Source: CAD feature listing. Evaluate the final solid. Frame: model axes, mm. A direction names the side the tool comes from. Give positions to 0.01 mm unless a question says otherwise; leave off trailing zeros. Loops run counter-clockwise (first coordinate to the right, second up) from the corner with the lowest first, then second, coordinate; pieces in that order, holes last. Notation, with made-up numbers: (59.5, 29.5) -> (94.5, 29.5) arc R21 cw to (94.5, 68.5) -> close; hole circle Ø11 at (-28.75, 51). An arc over 180 degrees is marked (long way). Return JSON: item names as keys, results as strings. Group by question number.
```python
from build123d import *

# Parameters (mm, degrees)
SKETCH1_R           = 2.159
SKETCH1_W           = 6.35
SKETCH1_H           = 6.35
BOSS_EXTRUDE1_DEPTH = 6.35


with BuildPart() as part:
    # Sketch1 → Boss-Extrude1 (new body)
    with BuildSketch(Plane(origin=(0, 0, 0), x_dir=(1, 0, 0), z_dir=(0, 1, 0))):
        Polygon((-25.4, 76.2), (-47.875911854, 76.2), (-60.633073629, 76.2), (-42.466090347, -115.062), (-22.93356755, -115.062), (-22.93356755, -120.142), (-41.98356755, -120.142), (-41.332161775, -127), (-28.575, -127), (0, -127), (28.575, -127), (41.332161775, -127), (60.633073629, 76.2), (47.875911854, 76.2), (25.4, 76.2), (25.4, 0), (13.208, 0), (13.208, 57.15), (6.858, 57.15), (6.858, 0), (-6.858, 0), (-6.858, 57.15), (-13.208, 57.15), (-13.208, 0), (-25.4, 0), align=None)
        Polygon((-39.17295277, -82.578452823), (-39.773403679, -76.256905647), (-33.451856503, -75.656454737), (-32.851405593, -81.978001914), align=None, mode=Mode.SUBTRACT)
        with Locations(Location((-37.41723431, -67.485806976, 0), (0, 0, 270))):
            Circle(SKETCH1_R, mode=Mode.SUBTRACT)
        Polygon((-35.66151585, -52.393161128), (-35.061064941, -58.714708304), (-41.382612117, -59.315159214), (-41.983063027, -52.993612037), align=None, mode=Mode.SUBTRACT)
        Polygon((29.83293553, -113.756454737), (36.154482707, -114.356905647), (35.554031797, -120.678452823), (29.232484621, -120.078001914), align=None, mode=Mode.SUBTRACT)
        with Locations(Location((33.798313337, -105.585806976, 0), (0, 0, 270))):
            Circle(SKETCH1_R, mode=Mode.SUBTRACT)
        Polygon((37.763691145, -97.415159214), (31.442143968, -96.814708304), (32.042594878, -90.493161128), (38.364142054, -91.093612037), align=None, mode=Mode.SUBTRACT)
        Polygon((-50.786897864, 39.693161128), (-51.387348774, 46.014708304), (-45.065801597, 46.615159214), (-44.465350687, 40.293612037), align=None, mode=Mode.SUBTRACT)
        with Locations((-34.925, 43.307)):
            Rectangle(SKETCH1_W, SKETCH1_H, mode=Mode.SUBTRACT)
        with Locations(Location((-49.031179404, 54.785806976, 0), (0, 0, 270))):
            Circle(SKETCH1_R, mode=Mode.SUBTRACT)
        Polygon((-47.275460944, 69.878452823), (-46.675010035, 63.556905647), (-52.996557211, 62.956454737), (-53.597008121, 69.278001914), align=None, mode=Mode.SUBTRACT)
        with Locations(Location((-34.925, 54.991, 0), (0, 0, 270))):
            Circle(SKETCH1_R, mode=Mode.SUBTRACT)
        with Locations((-34.925, 66.675)):
            Rectangle(SKETCH1_W, SKETCH1_H, mode=Mode.SUBTRACT)
        with Locations((34.925, 43.307)):
            Rectangle(SKETCH1_W, SKETCH1_H, mode=Mode.SUBTRACT)
        Polygon((45.065801597, 46.615159214), (51.387348774, 46.014708304), (50.786897864, 39.693161128), (44.465350687, 40.293612037), align=None, mode=Mode.SUBTRACT)
        with Locations(Location((34.925, 54.991, 0), (0, 0, 270))):
            Circle(SKETCH1_R, mode=Mode.SUBTRACT)
        with Locations((34.925, 66.675)):
            Rectangle(SKETCH1_W, SKETCH1_H, mode=Mode.SUBTRACT)
        with Locations(Location((49.031179404, 54.785806976, 0), (0, 0, 270))):
            Circle(SKETCH1_R, mode=Mode.SUBTRACT)
        Polygon((52.996557211, 62.956454737), (46.675010035, 63.556905647), (47.275460944, 69.878452823), (53.597008121, 69.278001914), align=None, mode=Mode.SUBTRACT)
    extrude(amount=BOSS_EXTRUDE1_DEPTH)


solid = part.part
```
1) Cut plane D-D on z = 16.5. Return loops of the section in (x, y).
2) Reachability of faces 5 (the face through (-22.934, 3, 118)), 6 (the face through (43, 3, -76.2)), 7 (the face through (-35, 3, -69.85)) from +Z, -Z, +X, -X, +Y, -Y: full face, straight path, thin tool, end or side. Return the list, or none.
3) Cut plane B-B on x = -21. Return loops of the section in (y, z).
4) Cut plane A-A on z = -10. Return loops of the section in (x, y), then the cut area to 3 significant figures.
5) Contact query for flat-ended pins moving along their axis: P1, Ø7, axis at x = -49.03, z = -54.79, coming from the -Y side; P2, Ø3, axis at y = 3, z = -42, coming from the +X side; P3, Ø3, axis at x = 19, y = 4, coming from the -Z side; P4, Ø3, axis at y = 3, z = -45, coming from the -X side. Output: stop coordinate, or through.
6) Material intervals for line 1 (Z direction, x = -24.5, y = 5.75); line 2 (X direction, y = 2.25, z = -23.5); line 3 (X direction, y = 4.75, z = -51), sorted ascending.
7) Cut plane C-C on y = 1. Count the separate pieces of the cut face and the enclosed holes in it, then the cut area to 3 significant figures.
8) Mould query, pull axis X, two halves, no side actions, for faces 1 (the face through (-47.6, 3.1, -56.4)), 2 (the face through (-1, 3, 127)), 3 (the face through (-41.662, 3.131, 123.523)), 4 (the face through (38.07, 3.13, 94.21)). Classes: released by +X, released by -X, zero draft, split by the parting line, or undercut.
Calculated:
{
 "1": {"outline": "(-51.83, 0) -> (51.83, 0) -> (51.83, 6.35) -> (-51.83, 6.35) -> close"},
 "2": {"face 5": "-X, +Y, -Y", "face 6": "-Z, +X, -X, +Y, -Y", "face 7": "+Y, -Y"},
 "3": {"outline": "(0, 0) -> (6.35, 0) -> (6.35, 127) -> (0, 127) -> close"},
 "4": {"outline": "(-54.35, 0) -> (-25.4, 0) -> (-25.4, 6.35) -> (-54.35, 6.35) -> close; (-13.21, 0) -> (-6.86, 0) -> (-6.86, 6.35) -> (-13.21, 6.35) -> close; (6.86, 0) -> (13.21, 0) -> (13.21, 6.35) -> (6.86, 6.35) -> close; (25.4, 0) -> (54.35, 0) -> (54.35, 6.35) -> (25.4, 6.35) -> close", "area": "448 mm2"},
 "5": {"P1": "y = 0", "P2": "x = 57.53", "P3": "z = 0", "P4": "x = -57.81"},
 "6": {"line 1": "0 to 115.06, 120.14 to 127", "line 2": "-55.63 to -25.4, -13.21 to -6.86, 6.86 to 13.21, 25.4 to 55.63", "line 3": "-58.24 to -25.4, -13.21 to -6.86, 6.86 to 13.21, 25.4 to 58.24"},
 "7": {"separate pieces": "1", "enclosed holes": "18", "area": "16,900 mm2"},
 "8": {"face 1": "undercut", "face 2": "zero draft", "face 3": "released by -X", "face 4": "undercut"}
}
